Model file for the job. Use its own axes, mm. Face numbers are marked on the shaded views. A direction names the side the tool comes from. Round coordinates to 2 decimals unless told otherwise and drop trailing zeros. Loops run counter-clockwise (first coordinate to the right, second up) from the corner with the lowest first, then second, coordinate; pieces in that order, holes last. Notation, with made-up numbers: (27.25, 46) - (86.25, 46) arc R23 cw to (86.25, 64) - close; hole circle Ø1 at (-29, 22). An arc over 180 degrees is marked (long way). Answer as a JSON object with one key per item and string values.
from build123d import *

# Parameters (mm, degrees)
F0_W     = 57.15
F0_H     = 31.75
F1_DEPTH = 38.1
F3_DEPTH = 12.7
F5_DEPTH = 12.7
F7_DEPTH = 25.401


with BuildPart() as f1:
    # F0 (on Front) → F1 (new body)
    with BuildSketch(Plane.XZ):
        with Locations((28.575, 15.875)):
            Rectangle(F0_W, F0_H)
    extrude(amount=F1_DEPTH)

    # F2 (on face) → F3 (cut)
    with BuildSketch(Plane.XZ.offset(38.1)):
        Polygon((57.15, 31.75), (19.05, 31.75), (31.75, 0), (57.15, 0), align=None)
    extrude(amount=-F3_DEPTH, mode=Mode.SUBTRACT)

    # F4 (on face) → F5 (cut)
    with BuildSketch(Plane(origin=(0, 0, 0), x_dir=(-1, 0, 0), z_dir=(0, 1, 0))):
        Polygon((-31.75, 0), (-19.05, 31.75), (-57.15, 31.75), (-57.15, 0), align=None)
    extrude(amount=-F5_DEPTH, mode=Mode.SUBTRACT)

    # F6 (on face) → F7 (cut, through all)
    with BuildSketch(Plane.XZ.offset(25.4)):
        Polygon((38.1, 31.75), (57.15, 0), (57.15, 31.75), align=None)
    extrude(amount=-F7_DEPTH, mode=Mode.SUBTRACT)


solid = f1.part
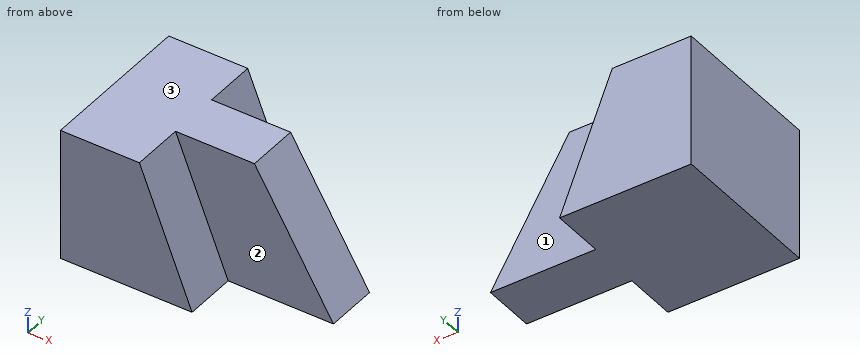
1) Slice it at D-D on x = 32.5. List the corners of the cut face in (y, z), then the cut area to 3 significant figures.
Values follow:
{"outline": "(-25.4, 0) - (-12.7, 0) - (-12.7, 31.75) - (-25.4, 31.75) - close", "area": "403 mm²"}
2) Slice it at C-C on y = -16. List the corners of the cut face in (x, z), then the cut area to 3 significant figures.
Values follow:
{"outline": "(0, 0) - (57.15, 0) - (38.1, 31.75) - (0, 31.75) - close", "area": "1,510 mm²"}
3) Tool access for the marked faces 1, 2 and 3: list every direction of +Z, -Z, +X, -X, +Y, -Y with a clear straight run to the whole face (end or side of a thin tool).
Values follow:
{"face 1": "+Z, +X, +Y", "face 2": "+Z, +X, -Y", "face 3": "+Z, +X, -X, +Y, -Y"}
4) Slice it at B-B on x = 24. List the corners of the cut face in (y, z) (3 decimals).
Values follow:
{"outline": "(-38.1, 0) - (0, 0) - (0, 19.375) - (-12.7, 19.375) - (-12.7, 31.75) - (-25.4, 31.75) - (-25.4, 19.375) - (-38.1, 19.375) - close"}
5) Drop flat-ended pins along their axis: P1, Ø6, axis at x = 32.5, y = -30, coming from the +Z side (3 decimals); P2, Ø4, axis at x = 48, z = 13.5, coming from the +Y side; P3, Ø5, axis at y = -10, z = 19, coming from the +X side. Give the stop position or say it passes through.
Values follow:
{"P1": "z = 5.625", "P2": "y = -12.7", "P3": "x = 25.15"}
6) Slice it at A-A on z = 9. List the corners of the cut face in (x, y), then the cut area to 3 significant figures.
Values follow:
{"outline": "(0, -38.1) - (28.15, -38.1) - (28.15, -25.4) - (51.75, -25.4) - (51.75, -12.7) - (28.15, -12.7) - (28.15, 0) - (0, 0) - close", "area": "1,370 mm²"}
7) Probe probe 1 along Y at (x, z) = (36, 6); probe 2 along X at (y, z) = (-10, 29.5); probe 3 along X at (y, z) = (-36, 26). List the from-to ranges inside material, lowest first.
Values follow:
{"probe 1": "-25.4 to -12.7", "probe 2": "0 to 19.95", "probe 3": "0 to 21.35"}
